from build123d import *

# Parameters (mm, degrees)
SKETCH3_W           = 13
SKETCH3_H           = 120
BOSS_EXTRUDE1_DEPTH = 4
SKETCH11_W          = 33
SKETCH11_H          = 120
BOSS_EXTRUDE4_DEPTH = 4
SKETCH12_R          = 2.5
CUT_EXTRUDE3_DEPTH  = 76.305579191
SKETCH13_W          = 6.102814475
SKETCH13_H          = 45
CUT_EXTRUDE4_DEPTH  = 76.305579191
SKETCH15_W          = 7.5
SKETCH15_H          = 6
CUT_EXTRUDE5_DEPTH  = 74.640547644


with BuildPart() as part:
    # Sketch3 → Boss-Extrude1 (new body)
    with BuildSketch(Plane.XY):
        with Locations((20.835766423, 0)):
            Rectangle(SKETCH3_W, SKETCH3_H)
        with BuildLine():
            Line((14.335766423, 0), (14.335766423, 60))
            Line((14.335766423, 60), (-22.664233577, 60))
            ThreePointArc((-22.664233577, 60), (-0.008037132, 46.062450015), (12.335766423, 22.5))
            Line((12.335766423, 22.5), (12.335766423, 0))
            Line((12.335766423, 0), (14.335766423, 0))
        make_face()
        with BuildLine():
            Line((14.335766423, -60), (14.335766423, 0))
            Line((14.335766423, 0), (12.335766423, 0))
            Line((12.335766423, 0), (12.335766423, -22.5))
            ThreePointArc((12.335766423, -22.5), (-0.008037132, -46.062450015), (-22.664233577, -60))
            Line((-22.664233577, -60), (14.335766423, -60))
        make_face()
    extrude(amount=BOSS_EXTRUDE1_DEPTH)


with BuildPart() as body_2:
    # Mirror4: mirrored copy
    add(part.part.mirror(Plane.XY.offset(-12.5)))


with BuildPart() as part_1:
    add(part.part)

    add(body_2.part)  # Boss-Extrude4 merges body 2
    # Sketch11 → Boss-Extrude4 (add)
    with BuildSketch(Plane(origin=(27.335766423, 0, 0), x_dir=(0, 0, -1), z_dir=(1, 0, 0))):
        with Locations((12.5, 0)):
            Rectangle(SKETCH11_W, SKETCH11_H)
    extrude(amount=BOSS_EXTRUDE4_DEPTH)

    # Sketch12 → Cut-Extrude3 (cut, through all)
    with BuildSketch(Plane.XY.offset(4)):
        with Locations((10.835766423, 52.5)):
            Circle(SKETCH12_R)
    cut_extrude3 = extrude(amount=-CUT_EXTRUDE3_DEPTH, mode=Mode.SUBTRACT)

    # Mirror5: Cut-Extrude3 across plane
    add(cut_extrude3.mirror(Plane.ZX), mode=Mode.SUBTRACT)

    # Sketch13 → Cut-Extrude4 (cut, through all)
    with BuildSketch(Plane.XY.offset(4)):
        with Locations((24.835766424, 0)):
            Rectangle(SKETCH13_W, SKETCH13_H)
    extrude(amount=-CUT_EXTRUDE4_DEPTH, mode=Mode.SUBTRACT)

    # Sketch15 → Cut-Extrude5 (cut, through all)
    with BuildSketch(Plane.XY.offset(-25)):
        with Locations((18.085766423, -38.5)):
            Rectangle(SKETCH15_W, SKETCH15_H)
    extrude(amount=-CUT_EXTRUDE5_DEPTH, mode=Mode.SUBTRACT)


solid = part_1.part
Check sheet for the modelled part. Datum: model origin and axes. Units: mm. A direction names the side the tool comes from. Give positions to 0.01 mm unless a question says otherwise; leave off trailing zeros. Loops run counter-clockwise (first coordinate to the right, second up) from the corner with the lowest first, then second, coordinate; pieces in that order, holes last. Notation, with made-up numbers: M 49.5,47 L 58.5,47 A21 cw 58.5,66 Z; hole C -19,60.25 d9. An arc over 180 degrees is marked long. Answer as a JSON object with one key per item and string values. Group by question number.
Q1. Go/stop test with flat-tipped pins: P1, Ø2, axis at y = -47, z = -9, coming from the -X side; P2, Ø4.5, axis at y = 2, z = 2, coming from the -X side; P3, Ø5, axis at x = 6, y = 28.5, coming from the -Z side; P4, Ø16.5, axis at y = 6.5, z = -8.5, coming from the -X side. Record where each tip stops, or that it passes through.
Q2. Cross-section at A-A on x = 18. Record the cut outline in (y, z), then the cut area to 3 significant figures.
Q3. Release check for a two-part mould opening along Y. For faces 5 (the flat face through (13, 1, -25)), 6 (the flat face through (21.784, 0, 2)) record: released by +Y, released by -Y, zero draft, split by the parting line, or undercut.
Q4. Cross-section at D-D on y = -52.5. Record the cut outline in (x, z).
Q5. Material ranges on line 1 along Z through (x, y) = (14, 10); line 2 along X through (y, z) = (-21.5, -26); line 3 along X through (y, z) = (-1, -1.5), recorded low to high. Write a range as [from, to].
Q6. Cross-section at C-C on z = -21.5. Record the cut outline in (x, y).
Q7. Cross-section at B-B on x = 24.5. Record the cut outline in (y, z).
Q8. Access from +Z, -Z, +X, -X, +Y, -Y to the whole of each face (thin tool, end or side, straight path). Record for faces 1 (the cylindrical face through (0.248, -45.786, -26.972)), 2 (the flat face through (18, -35.5, -27)), 3 (the flat face through (27.5, 22.5, -11.2)), 4 (the flat face through (27.336, 42, -12)).
Evaluation:
{
 "1": {"P1": "stops at x = 27.34", "P2": "stops at x = 12.34", "P3": "passes through", "P4": "stops at x = 27.89"},
 "2": {"outline": "M -60,-29 L -41.5,-29 L -41.5,-25 L -60,-25 Z; M -60,0 L 60,0 L 60,4 L -60,4 Z; M -35.5,-29 L 60,-29 L 60,-25 L -35.5,-25 Z", "area": "936 mm2"},
 "3": {"face 5": "zero draft", "face 6": "undercut"},
 "4": {"outline": "M -7.31,-29 L 8.34,-29 L 8.34,-25 L -7.31,-25 Z; M -7.31,0 L 8.34,0 L 8.34,4 L -7.31,4 Z; M 13.34,-29 L 31.34,-29 L 31.34,4 L 13.34,4 L 13.34,0 L 27.34,0 L 27.34,-25 L 13.34,-25 Z"},
 "5": {"line 1": "z = [-29, -25], [0, 4]", "line 2": "x = [12.34, 21.78], [27.89, 31.34]", "line 3": "x = [27.89, 31.34]"},
 "6": {"outline": "M 27.34,-60 L 31.34,-60 L 31.34,60 L 27.34,60 L 27.34,22.5 L 27.89,22.5 L 27.89,-22.5 L 27.34,-22.5 Z"},
 "7": {"outline": "M -60,-29 L -22.5,-29 L -22.5,-25 L -60,-25 Z; M -60,0 L -22.5,0 L -22.5,4 L -60,4 Z; M 22.5,-29 L 60,-29 L 60,-25 L 22.5,-25 Z; M 22.5,0 L 60,0 L 60,4 L 22.5,4 Z"},
 "8": {"face 1": "+Z, -Z, -X", "face 2": "-Z", "face 3": "+Z, -Z", "face 4": "-X, +Y, -Y"}
}
